```python
from build123d import *

# Parameters (mm, degrees)
BOSS_EXTRUDE1_DEPTH = 100
BOSS_EXTRUDE2_DEPTH = 20
SKETCH4_W           = 80
SKETCH4_H           = 31
BOSS_EXTRUDE3_DEPTH = 10
SKETCH4_2_W         = 80
SKETCH4_2_H         = 31
BOSS_EXTRUDE4_DEPTH = 20
SKETCH5_W           = 53
SKETCH5_H           = 22
SKETCH5_W_2         = 8
SKETCH5_H_2         = 18
CUT_EXTRUDE1_DEPTH  = 30
SKETCH6_W           = 10
SKETCH6_H           = 36
CUT_EXTRUDE2_DEPTH  = 80
SKETCH7_R           = 4.25
CUT_EXTRUDE3_DEPTH  = 162.012421881
CHAMFER1_SIZE       = 10


with BuildPart() as part:
    # Sketch1 → Boss-Extrude1 (new body)
    with BuildSketch(Plane.XY):
        Polygon((11, 0), (0, 0), (0, -10), (88, -10), (88, 0), (77, 0), (77, -3), (85, -3), (85, -7), (3, -7), (3, -3), (11, -3), align=None)
    extrude(amount=BOSS_EXTRUDE1_DEPTH)

    # Sketch2 → Boss-Extrude2 (add)
    with BuildSketch(Plane.XY.offset(100)):
        Polygon((77, 0), (11, 0), (11, -3), (3, -3), (3, -7), (85, -7), (85, -3), (77, -3), align=None)
        Polygon((4, 57), (4, 0), (11, 0), (77, 0), (84, 0), (84, 57), align=None)
        Polygon((0, 0), (0, -10), (88, -10), (88, 0), (84, 0), (77, 0), (77, -3), (85, -3), (85, -7), (3, -7), (3, -3), (11, -3), (11, 0), (4, 0), align=None)
    extrude(amount=BOSS_EXTRUDE2_DEPTH)

    # Sketch4 → Boss-Extrude3 (add)
    with BuildSketch(Plane.XY.offset(120)):
        with Locations((44, 5.5)):
            Rectangle(SKETCH4_W, SKETCH4_H)
    extrude(amount=BOSS_EXTRUDE3_DEPTH)

    # Sketch4<2> → Boss-Extrude4 (add)
    with BuildSketch(Plane.XY.offset(120)):
        with Locations((44, 5.5)):
            Rectangle(SKETCH4_2_W, SKETCH4_2_H)
    extrude(amount=-BOSS_EXTRUDE4_DEPTH)

    # Sketch5 → Cut-Extrude1 (cut)
    with BuildSketch(Plane.XY.offset(130)):
        with Locations((44, 7)):
            Rectangle(SKETCH5_W, SKETCH5_H)
        with Locations((8, 9)):
            Rectangle(SKETCH5_W_2, SKETCH5_H_2)
        with Locations((80, 9)):
            Rectangle(SKETCH5_W_2, SKETCH5_H_2)
    extrude(amount=-CUT_EXTRUDE1_DEPTH, mode=Mode.SUBTRACT)

    # Sketch6 → Cut-Extrude2 (cut)
    with BuildSketch(Plane.ZY.offset(-4)):
        with Locations((115, 39)):
            Rectangle(SKETCH6_W, SKETCH6_H)
    extrude(amount=-CUT_EXTRUDE2_DEPTH, mode=Mode.SUBTRACT)

    # Sketch7 → Cut-Extrude3 (cut, through all)
    with BuildSketch(Plane(origin=(76, 0, 0), x_dir=(0, 0, -1), z_dir=(1, 0, 0))):
        with Locations(Location((-122.7, 8.5, 0), (0, 0, 90))):
            Circle(SKETCH7_R)
    extrude(amount=-CUT_EXTRUDE3_DEPTH, mode=Mode.SUBTRACT)

    # Chamfer1
    chamfer1_edges = [part.edges().sort_by_distance(p)[0] for p in [
        (44, 21, 110),
    ]]
    chamfer(chamfer1_edges, length=CHAMFER1_SIZE)


solid = part.part
```
Input: part model. Units: mm. Frame: model coordinates. A direction names the side the tool comes from. Give positions to 0.01 mm unless a question says otherwise; leave off trailing zeros. Loops run counter-clockwise (first coordinate to the right, second up) from the corner with the lowest first, then second, coordinate; pieces in that order, holes last.
1) Line query: L1, parallel to Y at x = 6, z = 10; L2, parallel to Z at x = 74.35, y = 8.5; L3, parallel to X at y = -1, z = 48. Output: solid intervals per line, ascending.
A:
L1: y = -10 to -7, -3 to 0
L2: z = 100 to 118.45, 126.95 to 130
L3: x = 0 to 11, 77 to 88
2) Reachability of faces 4 (the flat face through (43, 21, 125)), 5 (the flat face through (12, 9, 115)), 6 (the flat face through (7, -3, 49)) from +Z, -Z, +X, -X, +Y, -Y: full face, straight path, thin tool, end or side. Return the list, or none.
A:
face 4: +Z, +X, -X, +Y
face 5: +Z, -Z, -X
face 6: -Z
3) Section query B-B on z = 122.7. Return the cut outline in (x, y).
A:
outline: (4, -10) - (84, -10) - (84, 0) - (76, 0) - (76, 4.25) - (70.5, 4.25) - (70.5, -4) - (17.5, -4) - (17.5, 4.25) - (12, 4.25) - (12, 0) - (4, 0) - close; (4, 18) - (12, 18) - (12, 12.75) - (17.5, 12.75) - (17.5, 18) - (70.5, 18) - (70.5, 12.75) - (76, 12.75) - (76, 18) - (84, 18) - (84, 21) - (4, 21) - close
4) Mould query, pull axis Y, two halves, no side actions, for faces 1 (the flat face through (43, -10, 64)), 2 (the flat face through (2, -5, 120)), 3 (the cylindrical face through (73.29, 5.13, 120.11)). Classes: released by +Y, released by -Y, zero draft, split by the parting line, or undercut.
A:
face 1: released by -Y
face 2: zero draft
face 3: undercut
5) Section query A-A on x = 20. Return the cut outline in (y, z), and give its area (3 significant figures).
A:
outline: (-10, 0) - (-7, 0) - (-7, 100) - (-4, 100) - (-4, 130) - (-10, 130) - close; (18, 100) - (57, 100) - (57, 110) - (31, 110) - (21, 120) - (21, 130) - (18, 130) - close
area: 980 mm2
6) Contact query for flat-ended pins moving along their axis: pin 1 (17.5 mm diameter, centred on y = 10, z = 120.5, fed in from -X); pin 2 (8 mm diameter, centred on x = 33.5, y = 3.5, fed in from -Z); pin 3 (2 mm diameter, centred on x = 86.5, y = -5, fed in from +Z); pin 4 (3 mm diameter, centred on y = 4.5, z = 102.5, fed in from -X). Output: stop coordinate, or through.
A:
pin 1: stops at x = 4
pin 2: passes through
pin 3: stops at z = 120
pin 4: stops at x = 12
7) Section query D-D on z = 42. Return the cut outline in (x, y), and give its area (3 significant figures).
A:
outline: (0, -10) - (88, -10) - (88, 0) - (77, 0) - (77, -3) - (85, -3) - (85, -7) - (3, -7) - (3, -3) - (11, -3) - (11, 0) - (0, 0) - close
area: 354 mm2
8) Section query C-C on y = 8.5. Return the cut outline in (x, z), and give its area (4 significant figures).
A:
outline: (12, 100) - (17.5, 100) - (17.5, 118.45) - (12, 118.45) - close; (12, 126.95) - (17.5, 126.95) - (17.5, 130) - (12, 130) - close; (70.5, 100) - (76, 100) - (76, 118.45) - (70.5, 118.45) - close; (70.5, 126.95) - (76, 126.95) - (76, 130) - (70.5, 130) - close
area: 236.5 mm2
